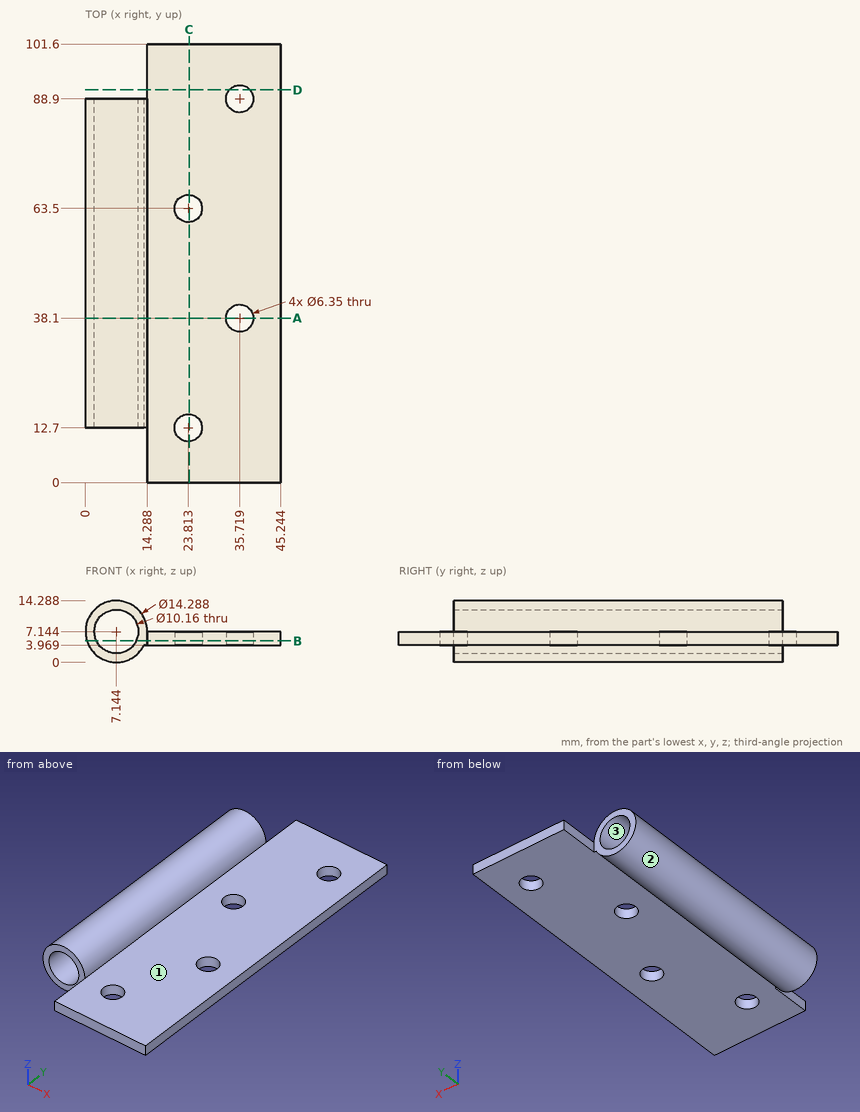
Design review of the part shown in the three views and the two pictorial views. Dimensions are in mm from the part's minimum x, y and z. Coordinates: 2 decimals unless noted, no trailing zeros. Loops run counter-clockwise (first coordinate to the right, second up) from the corner with the lowest first, then second, coordinate; pieces in that order, holes last. Notation, with made-up numbers: (45, 26.5) - (61, 26.5) arc R14 cw to (61, 39.5) - close; hole circle Ø6 at (86.25, 79.25). An arc over 180 degrees is marked (long way). Use a Markdown table: item, result. Add a question column.
Item 1: Insertion check: pin 1 Ø9.5 at (x, y) = (36.5, 65.5) entering from +Z; pin 2 Ø1 at (y, z) = (92, 6) entering from -X; pin 3 Ø7.5 at (x, y) = (23.81, 12.7) entering from -Z; pin 4 Ø4 at (x, y) = (35.72, 38.1) entering from -Z. Each pin has a flat end and moves straight along its axis. Give the tip position at first contact, or say it passes through.
Item 2: We need section A-A (y = 38.1). Give the boundary of the cut face in (x, z), and give its area (3 significant figures).
Item 3: Mouldability with a two-part tool opening along Z and no side actions: class the marked faces 1, 2 and 3 as pulls with the +Z half, pulls with the -Z half, needs draft (parallel to the pull), parting line crosses it, or undercut.
Item 4: We need section C-C (x = 24). Give the boundary of the cut face in (y, z).
Item 5: We need section D-D (y = 91). Give the boundary of the cut face in (x, z).
Item 6: For line 1 (Y direction, x = 24.5, z = 5.25); line 2 (Y direction, x = 26.5, z = 5.25); line 3 (X direction, y = 46.5, z = 9.25) (1 decimal), list the stretches that pass through material, from the lowest coordinate up.
Item 7: We need section B-B (z = 5). Give the number of separate pieces and of enclosed holes in the cut face, and give its area (3 significant figures).
Results list:
| question | item | result |
|---|---|---|
| 1 | pin 1 | stops at z = 7.14 |
| 1 | pin 2 | stops at x = 14.29 |
| 1 | pin 3 | stops at z = 3.97 |
| 1 | pin 4 | passes through |
| 2 | outline | (13.54, 3.97) - (32.54, 3.97) - (32.54, 7.14) - (14.29, 7.14) arc R7.14 ccw (long way) to start; (38.89, 3.97) - (45.24, 3.97) - (45.24, 7.14) - (38.89, 7.14) - close; hole circle Ø10.16 at (7.14, 7.14) |
| 2 | area | 158 mm^2 |
| 3 | face 1 | pulls with the +Z half |
| 3 | face 2 | parting line crosses it |
| 3 | face 3 | undercut |
| 4 | outline | (0, 3.97) - (9.53, 3.97) - (9.53, 7.14) - (0, 7.14) - close; (15.87, 3.97) - (60.33, 3.97) - (60.33, 7.14) - (15.87, 7.14) - close; (66.67, 3.97) - (101.6, 3.97) - (101.6, 7.14) - (66.67, 7.14) - close |
| 5 | outline | (14.29, 3.97) - (33.34, 3.97) - (33.34, 7.14) - (14.29, 7.14) - close; (38.1, 3.97) - (45.24, 3.97) - (45.24, 7.14) - (38.1, 7.14) - close |
| 6 | line 1 | y = 0 to 9.6, 15.8 to 60.4, 66.6 to 101.6 |
| 6 | line 2 | y = 0 to 11.01, 14.39 to 61.81, 65.19 to 101.6 |
| 6 | line 3 | x = 0.3 to 2.5, 11.8 to 14 |
| 7 | separate pieces | 2 |
| 7 | enclosed holes | 4 |
| 7 | area | 3,380 mm^2 |
